Source: CAD feature listing. Evaluate the final solid. Frame: model axes, mm. A direction names the side the tool comes from. Give positions to 0.01 mm unless a question says otherwise; leave off trailing zeros. Loops run counter-clockwise (first coordinate to the right, second up) from the corner with the lowest first, then second, coordinate; pieces in that order, holes last. Notation, with made-up numbers: M 87.5,-29.5 L 140.5,-29.5 A35 cw 140.5,2.5 Z; hole C 57.5,29 d2. An arc over 180 degrees is marked long. Put each result on its own line as item: value. Start each with the question number.
```python
from build123d import *

# Parameters (mm, degrees)
SKETCH_2_W          = 100
SKETCH_2_H          = 70
EXTRUDE_1_DEPTH     = 450
SKETCH_3_W          = 76
SKETCH_3_H          = 46
CUT_EXTRUDE_1_DEPTH = 420
SKETCH_4_W          = 76
SKETCH_4_H          = 46
CUT_EXTRUDE_2_DEPTH = 30
FILLET_1_R          = 8
FILLET_3_R          = 8


with BuildPart() as part:
    # 草图2 → 凸台-拉伸1 (new body)
    with BuildSketch(Plane.XY):
        Rectangle(SKETCH_2_W, SKETCH_2_H)
    extrude(amount=EXTRUDE_1_DEPTH)

    # 草图3 → 切除-拉伸1 (cut)
    with BuildSketch(Plane(origin=(0, 0, 0), x_dir=(-1, 0, 0), z_dir=(0, 0, -1))):
        Rectangle(SKETCH_3_W, SKETCH_3_H)
    extrude(amount=-CUT_EXTRUDE_1_DEPTH, mode=Mode.SUBTRACT)

    # 草图4 → 切除-拉伸2 (cut)
    with BuildSketch(Plane.XY.offset(450)):
        Rectangle(SKETCH_4_W, SKETCH_4_H)
    extrude(amount=-CUT_EXTRUDE_2_DEPTH, mode=Mode.SUBTRACT)

    # 圆角1
    fillet_1_edges = [part.edges().sort_by_distance(p)[0] for p in [
        (50, 0, 0),
    ]]
    fillet(fillet_1_edges, radius=FILLET_1_R)

    # 圆角3
    fillet_3_edges = [part.edges().sort_by_distance(p)[0] for p in [
        (-50, 0, 450),
    ]]
    fillet(fillet_3_edges, radius=FILLET_3_R)


solid = part.part
```
1. Section C-C, the plane x = 16. Output: boundary loops of the cut face in (y, z).
2. Ray query, line 1 (X direction, y = 5.5, z = 84); line 2 (Y direction, x = -20, z = 140); line 3 (Z direction, x = -44.5, y = 7). Return the intervals inside material, ascending.
3. Section B-B, the plane z = 33.5. Output: boundary loops of the cut face in (x, y), plus the area to 3 significant figures.
4. Pull-direction query (Y, two-part tool) for faces 1 (the face through (1, 23, 222)), 2 (the face through (1, -23, 222)), 3 (the face through (14, 24, 450)), 4 (the face through (-1, 35, 222)); classes: released by +Y, released by -Y, zero draft, split by the parting line, or undercut.
5. Section A-A, the plane y = -16.5. Output: boundary loops of the cut face in (x, z), plus the area to 3 significant figures.
6. Set-up query: faces 5 (the face through (-38, 0, 222)), 6 (the face through (-1, -35, 222)). Return all of +Z, -Z, +X, -X, +Y, -Y with unobstructed straight access to the full face (end or side cutting, diameter ignored); none if empty.
Results found:
1. outline: M -35,0 L -23,0 L -23,450 L -35,450 Z; M 23,0 L 35,0 L 35,450 L 23,450 Z
2. line 1: -50 to -38, 38 to 50
2. line 2: -35 to -23, 23 to 35
2. line 3: 0 to 449.6
3. outline: M -50,-35 L 50,-35 L 50,35 L -50,35 Z; hole M -38,-23 L 38,-23 L 38,23 L -38,23 Z
3. area: 3,500 mm²
4. face 1: undercut
4. face 2: undercut
4. face 3: zero draft
4. face 4: released by +Y
5. outline: M -50,0 L -38,0 L -38,450 L -42,450 A8 ccw -50,442 Z; M 38,0 L 42,0 A8 ccw 50,8 L 50,450 L 38,450 Z
5. area: 10,800 mm²
6. face 5: +Z, -Z
6. face 6: +Z, -Z, +X, -X, -Y
